Can you work these out from the drawing? Everything is in mm from the part's minimum corner. Give positions to 0.01 mm unless a question says otherwise; leave off trailing zeros. Loops run counter-clockwise (first coordinate to the right, second up) from the corner with the lowest first, then second, coordinate; pieces in that order, holes last. Notation, with made-up numbers: (45, 51.5) - (91, 51.5) arc R19 ccw to (91, 79.5) - close; hole circle Ø11 at (26, -17). An arc over 180 degrees is marked (long way). Write each question's results on one line, items separated by ' | '. Start each with the question number.
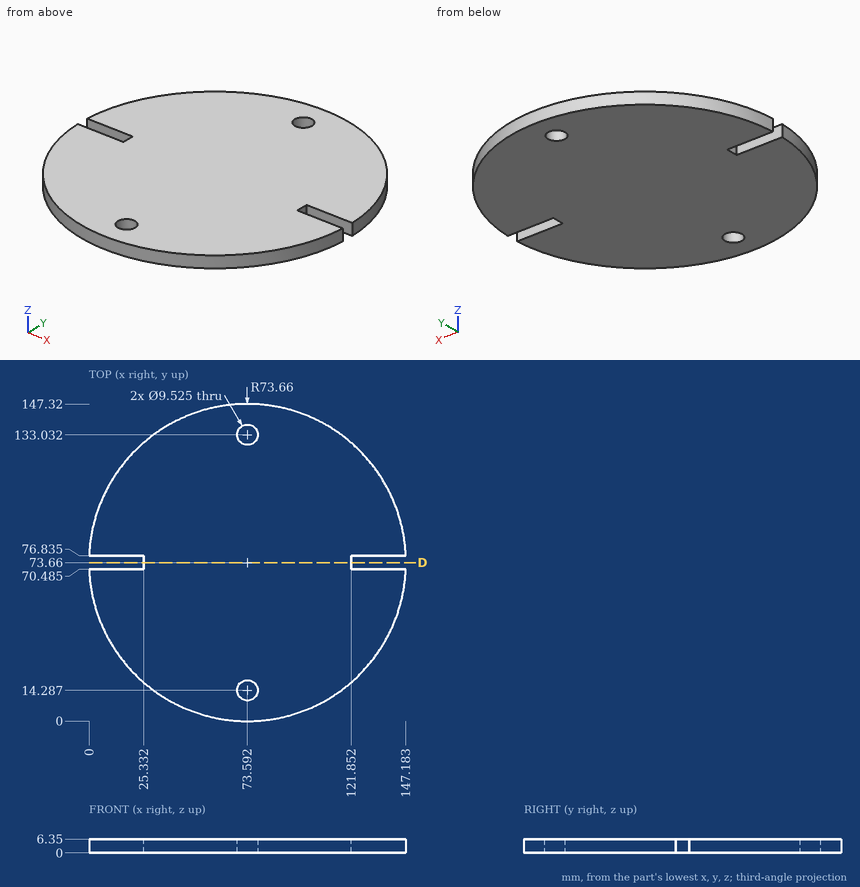
Q1. I need wall thicknesses on L1, parallel to Y at x = 73, z = 0.5; L2, parallel to Y at x = 11.5, z = 5.5 (1 decimal); L3, parallel to Y at x = 14, z = 5.75 (1 decimal). Which ranges of each line are inside material? Lowest first, please. Write a range as from..to.
Q2. I want a section at D-D, the plane y = 73.66. List the corners of the cut face in (x, z) for me, then the cut area to 3 significant figures.
Q3. I'm going to push flat-ended pins straight in: pin 1 Ø1.5 at (y, z) = (69, 2) entering from -X (1 decimal); pin 2 Ø3 at (y, z) = (72.5, 2) entering from -X; pin 3 Ø1.9 at (x, z) = (131, 3) entering from +Y. Where does each tip first touch, or does it pass through?
Conclusion:
1) L1: 0..9.56, 19.01..128.31, 137.76..147.32 | L2: 34..70.5, 76.8..113.3 | L3: 30.4..70.5, 76.8..117
2) outline: (25.33, 0) - (121.85, 0) - (121.85, 6.35) - (25.33, 6.35) - close | area: 613 mm^2
3) pin 1: x = 0 | pin 2: x = 25.33 | pin 3: y = 120.97
